Geometry: final body of the model. Coordinates: model frame, mm. Coordinates: 2 decimals unless noted, no trailing zeros. Loops run counter-clockwise (first coordinate to the right, second up) from the corner with the lowest first, then second, coordinate; pieces in that order, holes last. Notation, with made-up numbers: (83, -7.75) - (137, -7.75) arc R14 cw to (137, -1.75) - close; hole circle Ø3 at (-15, -37). An arc over 180 degrees is marked (long way). Put each result on its own line as item: value. Start each with the question number.
1) Section D-D on z = 45. Output: boundary loops of the cut face in (x, y).
2) Material intervals for line 1 along X through (y, z) = (0.8, 157); line 2 along X through (y, z) = (-0.4, 211); line 3 along Z through (x, y) = (28.5, -0.2), sorted ascending. Write a range as from..to.
3) Section C-C on y = -0.5. Count the separate pieces of the cut face and the enclosed holes in it, and give its area (3 significant figures).
4) Contact query for flat-ended pins moving along their axis: pin 1 Ø4 at (x, z) = (245.68, 11.29) entering from -Y; pin 2 Ø1.6 at (x, y) = (164, 0) entering from +Z; pin 3 Ø1 at (y, z) = (0, 160) entering from +X; pin 4 Ø1.6 at (y, z) = (0, 191) entering from -X. Output: stop coordinate, or through.
5) Section B-B on z = 191. Output: boundary loops of the cut face in (x, y).
6) Section A-A on z = 137. Output: boundary loops of the cut face in (x, y), and give its area (3 significant figures).
```python
from build123d import *

# Parameters (mm, degrees)
SKETCH1_W           = 570.861
SKETCH1_H           = 3.175
BOSS_EXTRUDE1_DEPTH = 232.6
SKETCH7_R           = 3.302
CUT_EXTRUDE4_DEPTH  = 369.216527271
SKETCH6_W           = 50
SKETCH6_H           = 3.175
BOSS_EXTRUDE2_DEPTH = 3.175
LPATTERN1_COUNT     = 6
LPATTERN1_PITCH     = 93.98
SKETCH2_W           = 3.175
SKETCH2_H           = 101.6
CUT_EXTRUDE5_DEPTH  = 371.230335845
BOSS_EXTRUDE3_DEPTH = 3.175
SKETCH13_W          = 3.175
SKETCH13_H          = 101.6
CUT_EXTRUDE6_DEPTH  = 396.22575932
LPATTERN2_COUNT     = 5
LPATTERN2_PITCH     = 91.9550104


with BuildPart() as part:
    # Sketch1 → Boss-Extrude1 (new body)
    with BuildSketch(Plane.XY):
        Rectangle(SKETCH1_W, SKETCH1_H)
    extrude(amount=BOSS_EXTRUDE1_DEPTH)

    # Sketch7 → Cut-Extrude4 (cut, through all)
    with BuildSketch(Plane(origin=(0, -1.5875, 0), x_dir=(-1, 0, 0), z_dir=(0, -1, 0))):
        with Locations(Location((-245.6805, -11.29165, 0), (0, 0, 90))):
            Circle(SKETCH7_R)
    cut_extrude4 = extrude(amount=-CUT_EXTRUDE4_DEPTH, mode=Mode.SUBTRACT)

    # Sketch6 → Boss-Extrude2 (add)
    with BuildSketch(Plane.XY.offset(232.6)):
        with Locations((127.26300405, 0)):
            Rectangle(SKETCH6_W, SKETCH6_H)
        with Locations((-55.6950692, 0)):
            Rectangle(SKETCH6_W, SKETCH6_H)
    extrude(amount=BOSS_EXTRUDE2_DEPTH)

    # LPattern1: Cut-Extrude4 ×6
    with Locations(*[(-i * LPATTERN1_PITCH, 0, 0) for i in range(1, LPATTERN1_COUNT)]):
        add(cut_extrude4, mode=Mode.SUBTRACT)

    # Sketch2 → Cut-Extrude5 (cut, through all)
    with BuildSketch(Plane(origin=(0, 1.5875, 0), x_dir=(1, 0, 0), z_dir=(0, 1, 0))):
        with Locations((-283.843, -50.8)):
            Rectangle(SKETCH2_W, SKETCH2_H)
        with Locations((283.843, -50.8)):
            Rectangle(SKETCH2_W, SKETCH2_H)
    extrude(amount=-CUT_EXTRUDE5_DEPTH, mode=Mode.SUBTRACT)

    # Sketch12 → Boss-Extrude3 (add)
    with BuildSketch(Plane(origin=(0, 1.5875, 0), x_dir=(1, 0, 0), z_dir=(0, 1, 0))):
        Polygon((-317.1805, -232.6), (-285.4305, -232.6), (-285.4305, -181.8), (-317.1805, -229.425), align=None)
    boss_extrude3 = extrude(amount=-BOSS_EXTRUDE3_DEPTH)

    # Mirror1: Boss-Extrude3 across plane
    add(boss_extrude3.mirror(Plane(origin=(0, 0, 0), x_dir=(0, 0, 1), z_dir=(1, 0, 0))))

    # Sketch13 → Cut-Extrude6 (cut, through all)
    with BuildSketch(Plane.XZ.offset(1.5875)):
        with Locations((-191.8879896, 181.8)):
            Rectangle(SKETCH13_W, SKETCH13_H)
    cut_extrude6 = extrude(amount=-CUT_EXTRUDE6_DEPTH, mode=Mode.SUBTRACT)

    # LPattern2: Cut-Extrude6 ×5
    with Locations(*[(i * LPATTERN2_PITCH, 0, 0) for i in range(1, LPATTERN2_COUNT)]):
        add(cut_extrude6, mode=Mode.SUBTRACT)


solid = part.part
```
Answer block:
1. outline: (-282.26, -1.59) - (282.26, -1.59) - (282.26, 1.59) - (-282.26, 1.59) - close
2. line 1: x = -285.43..-193.48, -190.3..-101.52, -98.35..-9.57, -6.39..82.39, 85.56..174.34, 177.52..285.43
2. line 2: x = -304.9..-193.48, -190.3..-101.52, -98.35..-9.57, -6.39..82.39, 85.56..174.34, 177.52..304.9
2. line 3: z = 0..232.6
3. separate pieces: 1
3. enclosed holes: 6
3. area: 132,000 mm²
4. pin 1: passes through
4. pin 2: stops at z = 232.6
4. pin 3: stops at x = 285.43
4. pin 4: stops at x = -292.1
5. outline: (-291.56, -1.59) - (-193.48, -1.59) - (-193.48, 1.59) - (-291.56, 1.59) - close; (-190.3, -1.59) - (-101.52, -1.59) - (-101.52, 1.59) - (-190.3, 1.59) - close; (-98.35, -1.59) - (-9.57, -1.59) - (-9.57, 1.59) - (-98.35, 1.59) - close; (-6.39, -1.59) - (82.39, -1.59) - (82.39, 1.59) - (-6.39, 1.59) - close; (85.56, -1.59) - (174.34, -1.59) - (174.34, 1.59) - (85.56, 1.59) - close; (177.52, -1.59) - (291.56, -1.59) - (291.56, 1.59) - (177.52, 1.59) - close
6. outline: (-285.43, -1.59) - (-193.48, -1.59) - (-193.48, 1.59) - (-285.43, 1.59) - close; (-190.3, -1.59) - (-101.52, -1.59) - (-101.52, 1.59) - (-190.3, 1.59) - close; (-98.35, -1.59) - (-9.57, -1.59) - (-9.57, 1.59) - (-98.35, 1.59) - close; (-6.39, -1.59) - (82.39, -1.59) - (82.39, 1.59) - (-6.39, 1.59) - close; (85.56, -1.59) - (174.34, -1.59) - (174.34, 1.59) - (85.56, 1.59) - close; (177.52, -1.59) - (285.43, -1.59) - (285.43, 1.59) - (177.52, 1.59) - close
6. area: 1,760 mm²
